```python
from build123d import *

# Parameters (mm, degrees)
F1_DEPTH = 25.4
F2_W     = 25.360864
F2_H     = 25.4
F3_DEPTH = 12.7


with BuildPart() as f1:
    # F0 (on Right) → F1 (new body)
    with BuildSketch(Plane.YZ):
        Polygon((0, 6.35), (0, 0), (25.4, 0), (25.4, 19.05), (19.05, 19.05), (19.05, 6.35), align=None)
    extrude(amount=F1_DEPTH)

    # F2 (on Right) → F3 (join)
    with BuildSketch(Plane.YZ):
        with Locations((12.680432, 12.7)):
            Rectangle(F2_W, F2_H)
    extrude(amount=-F3_DEPTH)


solid = f1.part
```
CAD build for the part. Positions are in the model's coordinates, mm. A direction names the side the tool comes from. Round coordinates to 2 decimals unless told otherwise and drop trailing zeros. Write each loop counter-clockwise with the first axis right and the second up, starting at its lowest first coordinate (ties: lowest second). Pieces come first, ordered by that corner, then holes.
Item 1: Tool access for faces 1 (the flat face through (13, 22, 19.05)), 2 (the flat face through (13, 19.05, 13)), 3 (the flat face through (-6, 25.361, 13)): list every direction of +Z, -Z, +X, -X, +Y, -Y with a clear straight run to the whole face (end or side of a thin tool).
Filled in:
face 1: +Z, +X, +Y, -Y
face 2: +Z, +X, -Y
face 3: +Z, -Z, -X, +Y
Item 2: Band-saw the part on D-D on z = 20. Write the cut outline in (x, y), then the cut area to 3 significant figures.
Filled in:
outline: (-12.7, 0) - (0, 0) - (0, 25.36) - (-12.7, 25.36) - close
area: 322 mm2
Item 3: Drill centre lines: L1, parallel to X at y = 20.25, z = 23.5; L2, parallel to Z at x = 1.5, y = 11.25; L3, parallel to Y at x = -2, z = 9.5. Where is each one in solid material? Low to high.
Filled in:
L1: x = -12.7 to 0
L2: z = 0 to 6.35
L3: y = 0 to 25.36
Item 4: Drop flat-ended pins along their axis: pin 1 Ø3 at (x, y) = (20.5, 17.5) entering from +Z; pin 2 Ø5 at (x, y) = (18.5, 21.5) entering from +Z; pin 3 Ø10 at (x, z) = (8.5, 12) entering from -Y. Give the stop position or say it passes through.
Filled in:
pin 1: stops at z = 6.35
pin 2: stops at z = 19.05
pin 3: stops at y = 19.05
Item 5: Band-saw the part on A-A on y = 6.25. Write the cut outline in (x, z).
Filled in:
outline: (-12.7, 0) - (25.4, 0) - (25.4, 6.35) - (0, 6.35) - (0, 25.4) - (-12.7, 25.4) - close
Item 6: Band-saw the part on C-C on x = 12. Write the cut outline in (y, z), then the cut area to 3 significant figures.
Filled in:
outline: (0, 0) - (25.4, 0) - (25.4, 19.05) - (19.05, 19.05) - (19.05, 6.35) - (0, 6.35) - close
area: 242 mm2
